Source: three-view drawing plus pictorial views. Frame: mm from the lowest corner of the part. Round coordinates to 2 decimals unless told otherwise and drop trailing zeros. Loops run counter-clockwise (first coordinate to the right, second up) from the corner with the lowest first, then second, coordinate; pieces in that order, holes last. Notation, with made-up numbers: (-27, 84) -> (27, 84) arc R28 ccw to (27, 107) -> close; hole circle Ø4 at (-9, 42.25). An arc over 180 degrees is marked (long way). Put each result on its own line as item: value. Start each with the question number.
1. Cut plane B-B (z = 2.95). State how many separate pieces and enclosed holes the cut face has, then the cut area to 3 significant figures.
2. Cut plane A-A (x = 242). Return the cut outline in (y, z), then the cut area to 3 significant figures.
3. Cut plane C-C (x = 42). Return the cut outline in (y, z).
4. Material intervals for L1, parallel to Y at x = 280, z = 1.75; L2, parallel to Y at x = 97, z = 2.9; L3, parallel to X at y = 75.5, z = 3.85, sorted ascending.
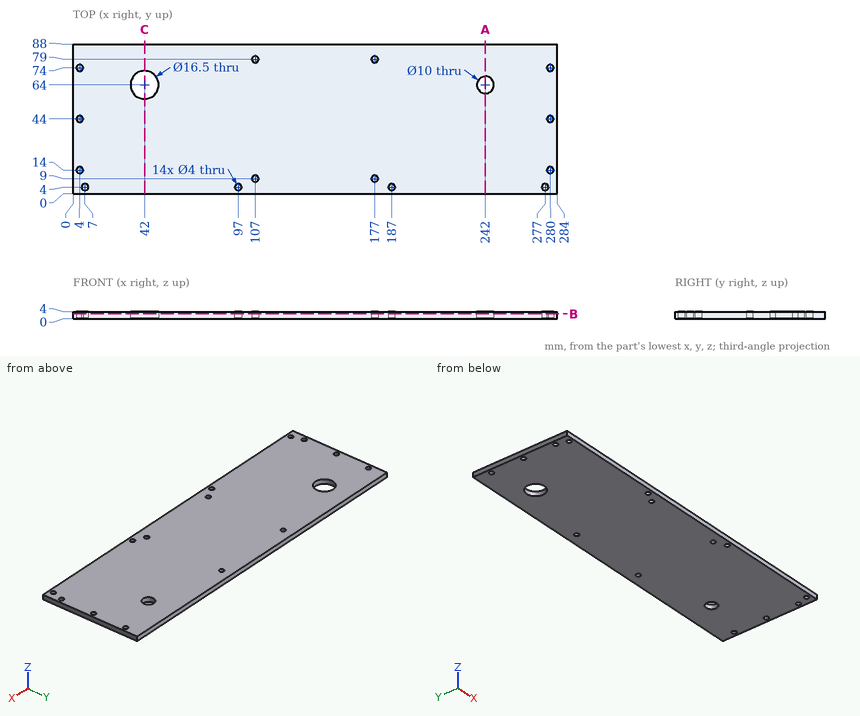
Solution:
1. separate pieces: 1
1. enclosed holes: 16
1. area: 24,500 mm^2
2. outline: (0, 0) -> (59, 0) -> (59, 4) -> (0, 4) -> close; (69, 0) -> (88, 0) -> (88, 4) -> (69, 4) -> close
2. area: 312 mm^2
3. outline: (0, 0) -> (55.75, 0) -> (55.75, 4) -> (0, 4) -> close; (72.25, 0) -> (88, 0) -> (88, 4) -> (72.25, 4) -> close
4. L1: y = 0 to 12, 16 to 42, 46 to 72, 76 to 88
4. L2: y = 0 to 2, 6 to 88
4. L3: x = 0 to 2.68, 5.32 to 278.68, 281.32 to 284
